Check sheet for the modelled part. Datum: model origin and axes. Units: mm. Face numbers are marked on the shaded views. A direction names the side the tool comes from. Give positions to 0.01 mm unless a question says otherwise; leave off trailing zeros. Loops run counter-clockwise (first coordinate to the right, second up) from the corner with the lowest first, then second, coordinate; pieces in that order, holes last. Notation, with made-up numbers: (85.25, 61) - (116.25, 61) arc R17 ccw to (116.25, 91) - close; hole circle Ø10 at (-4, 23). An arc over 180 degrees is marked (long way). Use CSV: the item, a comma, the result in double quotes.
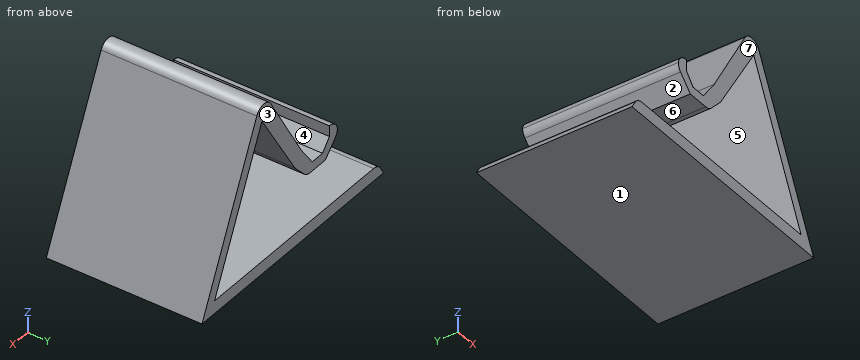
from build123d import *

# Parameters (mm, degrees)
F1_DEPTH    = 71.882
F2_R        = 5.08
F3_T1_DEPTH = 112.7375789557
F3_T3_DEPTH = 85.95990044
F3_T5_DEPTH = 120.1718750332
F3_T7_DEPTH = 82.9446926806


# Not quite as in the source:
# - a fillet or chamfer that OpenCascade refuses, or shapes differently, is made with other operations: its cross-section is extruded or revolved along the edge and cut away or added


with BuildPart() as f1:
    # F0 (on Front) → F1 (new body)
    with BuildSketch(Plane.XZ):
        Polygon((-35.8331985772, 9.4200642779), (-35.8331985772, 14.96128086), (-41.0050004721, 17.5471808761), (-41.0050004721, 7.9424064606), (-33.2472957671, 0), (-21.0566222668, 0), (-13.6683331802, 7.9424064606), (7.7815425405, 42.8511098702), (38.4191013873, -22.7189920843), (-67.233428359, -22.7189920843), (-70.92756778, -28.6296233535), (46.5462207794, -28.6296233535), (7.0188767277, 55.9662804008), (-17.7318900824, 13.8530377299), (-24.750765413, 4.2482619174), (-31.4002260566, 4.2482619174), align=None)
    extrude(amount=F1_DEPTH)

    # F2
    f2_edges = [f1.edges().sort_by_distance(p)[0] for p in [
        (-41.005, -35.941, 7.942406),
    ]]
    fillet(f2_edges, radius=F2_R)

    # F3: fillet of radius 5.08 on 4 edges, made by hand

    # F3_s2 → F3_t1 (cut)
    with BuildSketch(Plane.XZ.offset(-20.4277894779)):
        with BuildLine():
            ThreePointArc((-41.0050004721, 10.0116893284), (-38.3510310012, 13.8358325022), (-33.6965318012, 13.8929478568))
            Line((-33.6965318012, 13.8929478568), (-41.0050004721, 17.5471808761))
            Line((-41.0050004721, 17.5471808761), (-41.0050004721, 10.0116893284))
        make_face()
    extrude(amount=F3_T1_DEPTH, mode=Mode.SUBTRACT)

    # F3_s4 → F3_t3 (cut)
    with BuildSketch(Plane.XZ.offset(-7.03895022)):
        with BuildLine():
            ThreePointArc((-64.417848271, -22.7189920843), (-66.8804738001, -23.3558090469), (-68.7256813332, -25.1066001536))
            Line((-68.7256813332, -25.1066001536), (-67.233428359, -22.7189920843))
            Line((-67.233428359, -22.7189920843), (-64.417848271, -22.7189920843))
        make_face()
    extrude(amount=F3_T3_DEPTH, mode=Mode.SUBTRACT)

    # F3_s6 → F3_t5 (cut)
    with BuildSketch(Plane.XZ.offset(-24.1449375166)):
        with BuildLine():
            ThreePointArc((2.1252810988, 47.6398644221), (6.7441636939, 50.1402432188), (11.1072770532, 47.2163396005))
            Line((11.1072770532, 47.2163396005), (7.0188767277, 55.9662804008))
            Line((7.0188767277, 55.9662804008), (2.1252810988, 47.6398644221))
        make_face()
    extrude(amount=F3_T5_DEPTH, mode=Mode.SUBTRACT)

    # F3_s8 → F3_t7 (cut)
    with BuildSketch(Plane.XZ.offset(-5.5313463403)):
        with BuildLine():
            ThreePointArc((-23.2691608029, 0), (-21.2406694782, 0.4225733558), (-19.5496531088, 1.6199909663))
            Line((-19.5496531088, 1.6199909663), (-21.0566222668, 0))
            Line((-21.0566222668, 0), (-23.2691608029, 0))
        make_face()
    extrude(amount=F3_T7_DEPTH, mode=Mode.SUBTRACT)


solid = f1.part
1. Go/stop test with flat-tipped pins: pin 1 Ø2 at (x, y) = (-29, -30.5) entering from +Z; pin 2 Ø3 at (y, z) = (-19, 30) entering from +X; pin 3 Ø4 at (y, z) = (-43.5, 11.5) entering from +X. Record where each tip stops, or that it passes through.
Completed:
pin 1,"stops at z = 4.25"
pin 2,"stops at x = 19.85"
pin 3,"stops at x = 28.73"
2. Set-up check for the marked faces 4, 5, 6 and 7: record each of +Z, -Z, +X, -X, +Y, -Y from which the full face is reachable in a straight line by a thin tool's end or side.
Completed:
face 4,"+Z, +Y, -Y"
face 5,"+Y, -Y"
face 6,"-X, +Y, -Y"
face 7,"+Z, -Z, +X, -X, -Y"
3. Scan lines: line 1 along X through (y, z) = (-13, 11.5); line 2 along X through (y, z) = (-30.5, 39.5); line 3 along X through (y, z) = (-27, 9.5). Record each from-to range of solid material in increasing order.
Completed:
line 1,"x = -40.57 to -35.83, -19.45 to -11.48, 22.43 to 27.8"
line 2,"x = -2.66 to 5.72, 9.35 to 14.71"
line 3,"x = -40.98 to -35.83, -20.91 to -12.71, 23.36 to 28.73"
4. Release check for a two-part mould opening along Z. For the marked faces 1, 2 and 3 record: released by +Z, released by -Z, zero draft, split by the parting line, or undercut.
Completed:
face 1,"released by -Z"
face 2,"undercut"
face 3,"zero draft"
5. Sectioned sample at C-C, the plane y = -37. Record the boundary of the cut face in (x, z) (3 decimals), and give its area (3 significant figures).
Completed:
outline,"(-70.928, -28.63) - (46.546, -28.63) - (11.107, 47.216) arc R5.08 ccw to (2.125, 47.64) - (-17.732, 13.853) - (-24.751, 4.248) - (-31.4, 4.248) - (-35.833, 9.42) - (-35.833, 14.427) arc R5.08 ccw to (-41.005, 10.012) arc R5.08 ccw to (-39.559, 6.462) - (-33.247, 0) - (-23.269, 0) arc R5.08 ccw to (-19.55, 1.62) - (-13.668, 7.942) - (7.782, 42.851) - (38.419, -22.719) - (-64.418, -22.719) arc R5.08 ccw to (-68.726, -25.107) - close"
area,"1,530 mm²"
6. Sectioned sample at B-B, the plane x = 30. Record the boundary of the cut face in (y, z), and give its area (3 significant figures).
Completed:
outline,"(-71.88, -28.63) - (0, -28.63) - (0, -22.72) - (-71.88, -22.72) - close; (-71.88, -4.7) - (0, -4.7) - (0, 6.78) - (-71.88, 6.78) - close"
area,"1,250 mm²"
7. Sectioned sample at D-D, the plane z = 12. Record the boundary of the cut face in (x, y), and give its area (3 significant figures).
Completed:
outline,"(-40.3, -71.88) - (-35.83, -71.88) - (-35.83, 0) - (-40.3, 0) - close; (-19.09, -71.88) - (-11.18, -71.88) - (-11.18, 0) - (-19.09, 0) - close; (22.2, -71.88) - (27.56, -71.88) - (27.56, 0) - (22.2, 0) - close"
area,"1,280 mm²"
8. Sectioned sample at A-A, the plane z = 41. Record the boundary of the cut face in (x, y).
Completed:
outline,"(-1.78, -71.88) - (6.64, -71.88) - (6.64, 0) - (-1.78, 0) - close; (8.65, -71.88) - (14.01, -71.88) - (14.01, 0) - (8.65, 0) - close"
